Could you check a few things on this drawing? It's one solid part, dimensions in mm from its lowest x, y, z. A direction names the side the tool comes from. Give positions to 0.01 mm unless a question says otherwise; leave off trailing zeros. Loops run counter-clockwise (first coordinate to the right, second up) from the corner with the lowest first, then second, coordinate; pieces in that order, holes last.
1. Imagine slicing it at A-A (x = 25.4). List the corners of the cut face in (y, z) for me, plus the area to 3 significant figures.
2. I need wall thicknesses on line 1 along Y through (x, z) = (25.4, 0.85); line 2 along Y through (x, z) = (9.75, 10.25); line 3 along Z through (x, y) = (23.25, 1.25). Which ranges of each line are inside material? Lowest first, please.
3. For the marked faces 1, 2, 3 and 4, which set-ups out of +Z, -Z, +X, -X, +Y, -Y let a thin tool reach every point of the face, with its end or its side?
4. Imagine slicing it at C-C (y = 3.5). Count the separate pieces of the cut face and the enclosed holes in it, plus the area to 3 significant figures.
5. Thinking about a two-plate mould opening in Y: for the marked faces 5, 6 and 7, which applies, +Y half, -Y half, draft (parallel to the pull), parting line (faces both ways), or undercut?
6. For P1, Ø4, axis at x = 15, z = 13.5, coming from the -Y side; P2, Ø12, axis at x = 4, z = 2.5, coming from the -Y side; P3, Ø3.5, axis at x = 25.4, y = 3.175, coming from the +Z side; P4, Ø1.1, axis at y = 1.5, z = 20, coming from the -X side, each with a flat end and sliding along its axis, tell me the tip position at first contact or that it passes through.
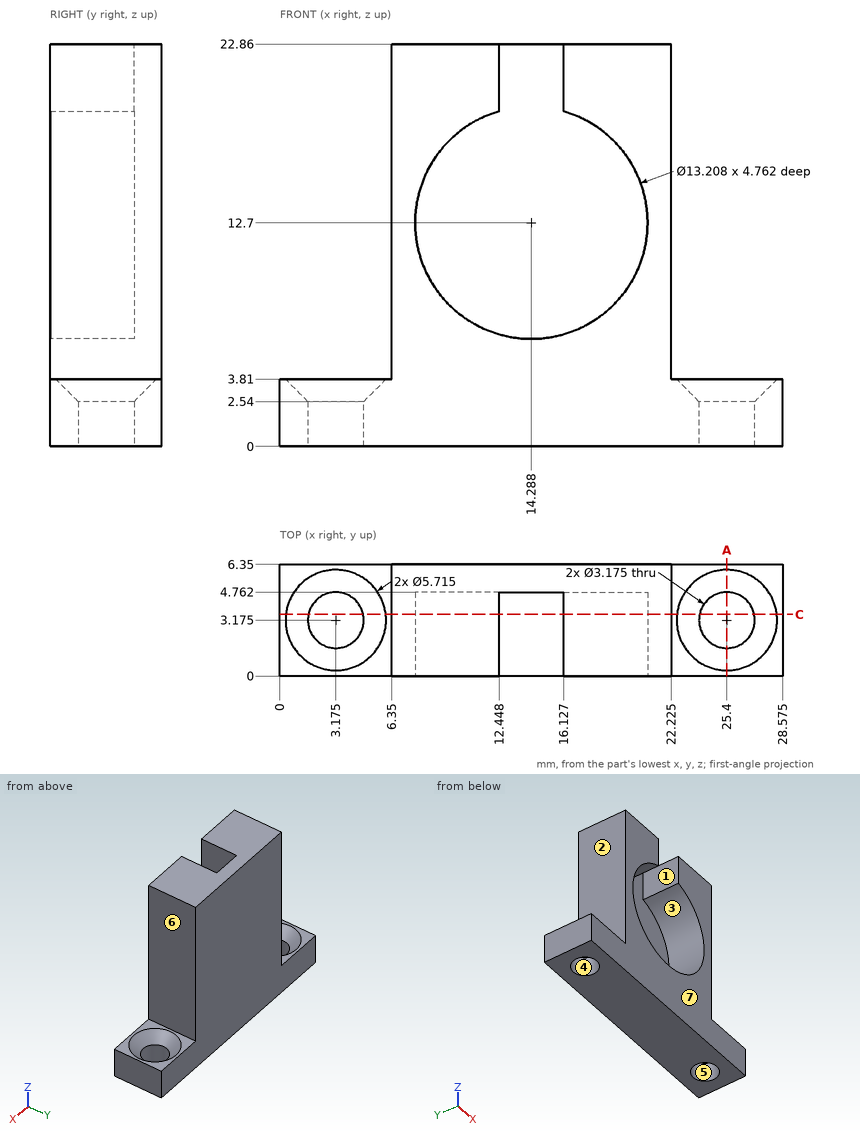
Derived:
1. outline: (0, 0) - (1.59, 0) - (1.59, 2.54) - (0.32, 3.81) - (0, 3.81) - close; (4.76, 0) - (6.35, 0) - (6.35, 3.81) - (6.03, 3.81) - (4.76, 2.54) - close
1. area: 10.5 mm2
2. line 1: y = 0 to 1.59, 4.76 to 6.35
2. line 2: y = 4.76 to 6.35
2. line 3: z = 0 to 3.81
3. face 1: +Z, -Y
3. face 2: +Z, -X, +Y, -Y
3. face 3: -Y
3. face 4: +Z, -Z
4. separate pieces: 3
4. enclosed holes: 0
4. area: 234 mm2
5. face 5: undercut
5. face 6: draft
5. face 7: -Y half
6. P1: stops at y = 4.76
6. P2: stops at y = 0
6. P3: stops at z = 2.7
6. P4: stops at x = 6.35
